Geometry check sheet. Reference: the model listing, model coordinates, mm. Coordinates: 2 decimals unless noted, no trailing zeros. Loops run counter-clockwise (first coordinate to the right, second up) from the corner with the lowest first, then second, coordinate; pieces in that order, holes last.
from build123d import *

# Parameters (mm, degrees)
F1_DEPTH = 3
F2_W     = 12
F2_H     = 56
F3_DEPTH = 3
F4_D     = 3
F6_D     = 2


with BuildPart() as f1:
    # F0 (on Top) → F1 (new body)
    with BuildSketch(Plane.XY):
        Polygon((-78.133352, 32.29949), (-93.133352, 32.29949), (-93.133352, -17.70051), (-78.133352, -17.70051), (-78.133352, -20.70051), (-66.133352, -20.70051), (-66.133352, -17.70051), (-20.133352, -17.70051), (-20.133352, -20.70051), (-8.133352, -20.70051), (-8.133352, -17.70051), (6.866648, -17.70051), (6.866648, 32.29949), (-8.133352, 32.29949), (-8.133352, 35.29949), (-20.133352, 35.29949), (-20.133352, 32.29949), (-66.133352, 32.29949), (-66.133352, 35.29949), (-78.133352, 35.29949), align=None)
    extrude(amount=F1_DEPTH)

    # F2 (on face) → F3 (join)
    with BuildSketch(Plane.XY.offset(3)):
        Polygon((-78.133352, 35.29949), (-78.133352, 32.29949), (-78.133352, -17.70051), (-78.133352, -20.70051), (-66.133352, -20.70051), (-66.133352, -17.70051), (-66.133352, 35.29949), align=None)
        with Locations((-14.133352, 7.29949)):
            Rectangle(F2_W, F2_H)
    extrude(amount=F3_DEPTH)

    # F4 (through all)
    with Locations(Plane.XY.offset(3)):
        with Locations((-90.133352, -14.70051), (-90.133352, 29.29949), (3.866648, -14.70051), (3.866648, 29.29949)):
            Hole(F4_D / 2)

    # F6 (through all)
    with Locations(Plane.XY.offset(3)):
        with Locations((-53.966256, 19.074386), (-43.133352, 23.29949), (-32.300447, 19.074386), (-27.133352, 7.29949), (-32.300447, -4.475406), (-34.331617, -2.267613), (-36.362787, -0.05982), (-38.393956, 2.147973), (-40.425126, 4.355766), (-39.133352, 7.29949), (-36.133352, 7.29949), (-33.133352, 7.29949), (-30.133352, 7.29949), (-40.425126, 10.243214), (-38.393956, 12.451007), (-36.362787, 14.6588), (-34.331617, 16.866593), (-43.133352, 11.29949), (-43.133352, 14.29949), (-43.133352, 17.29949), (-43.133352, 20.29949), (-51.935087, 16.866593), (-49.903917, 14.6588), (-47.872748, 12.451007), (-45.841578, 10.243214), (-47.133352, 7.29949), (-45.841578, 4.355766), (-43.133352, 3.29949), (-43.133352, 0.29949), (-43.133352, -2.70051), (-43.133352, -5.70051), (-43.133352, -8.70051), (-53.966256, -4.475406), (-51.935087, -2.267613), (-49.903917, -0.05982), (-47.872748, 2.147973), (-50.133352, 7.29949), (-53.133352, 7.29949), (-56.133352, 7.29949), (-59.133352, 7.29949), (-43.133352, 7.29949)):
            Hole(F6_D / 2)


solid = f1.part
1) Material ranges on probe 1 along X at (y, z) = (-3, 2.8); probe 2 along Y at (x, z) = (-49.5, 1.15); probe 3 along X at (y, z) = (-13.5, 1.5), recorded low to high.
Data:
probe 1: x = -93.13 to -52.62, -51.25 to -44.09, -42.18 to -35.01, -33.65 to 6.87
probe 2: y = -17.7 to -0.97, 0.85 to 6.53, 8.07 to 13.74, 15.57 to 32.3
probe 3: x = -93.13 to -91.03, -89.23 to 2.97, 4.77 to 6.87
2) Depth check by flat-ended pin: pin 1 (2.5 mm diameter, centred on x = -30.13, y = 7.3, fed in from +Z); pin 2 (1 mm diameter, centred on x = -37.5, z = 2, fed in from +Y); pin 3 (2.5 mm diameter, centred on x = -45.5, z = 2, fed in from -Y). Enter the tip coordinate at first touch or a pass-through.
Data:
pin 1: stops at z = 3
pin 2: stops at y = 32.3
pin 3: stops at y = -17.7
3) Mould release check, pull along Y, two halves, no side actions. Record for faces 1 (the cylindrical face through (-42.4, 23.98, 1.48)), 2 (the flat face through (-72, -20.701, 3)), 3 (the flat face through (-78.133, 8, 4)), 4 (the flat face through (-72, 35.299, 3)): +Y half, -Y half, draft (parallel to the pull), parting line (faces both ways), or undercut.
Data:
face 1: undercut
face 2: -Y half
face 3: draft
face 4: +Y half
4) Section check B-B on z = 1.5. Count the separate pieces of the cut face and the enclosed holes in it, and give its area (3 significant figures).
Data:
separate pieces: 1
enclosed holes: 45
area: 4,990 mm2
5) Section check A-A on x = -3.5. Record the cut outline in (y, z), and give its area (3 significant figures).
Data:
outline: (-17.7, 0) - (32.3, 0) - (32.3, 3) - (-17.7, 3) - close
area: 150 mm2
